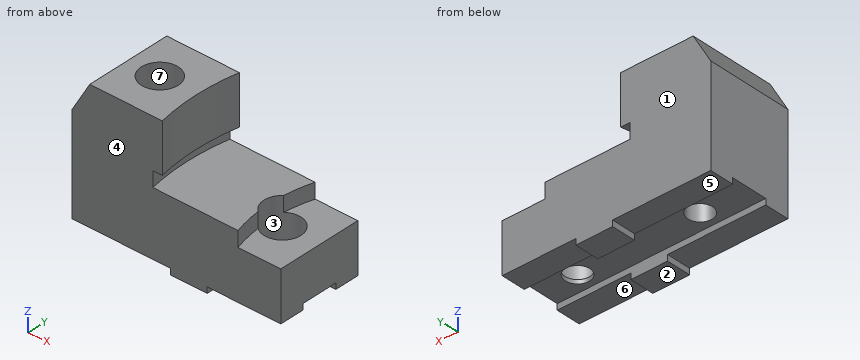
from build123d import *

# Parameters (mm, degrees)
F0_W                   = 107.95
F0_H                   = 69.85
F1_DEPTH               = 44.45
F2_W                   = 50.8254
F2_H                   = 3.048
F2_W_2                 = 38.1
F3_DEPTH               = 66.64201
F3_DEPTH_BACK          = 161
F4_W                   = 19.1008
F4_H                   = 3.048
F4_H_2                 = 17.1056788669
F5_DEPTH               = 107.951
F7_DEPTH               = 33.274
F9_W                   = 18.9599941809
F9_H                   = 7.874
F11_W                  = 28.8704986477
F11_H                  = 14.4021337534
F12_ANGLE_BACK         = 30
F12_ANGLE              = 60
F15_D                  = 12.7
F15_CBORE_D            = 19.05
F15_CBORE_DEPTH        = 20.574
F15_ON_F14_D           = 12.7
F15_ON_F14_START       = 7.874
F15_ON_F14_CBORE_D     = 19.05
F15_ON_F14_CBORE_DEPTH = 20.574


# Not quite as in the source:
# - an extrude ends at something that could not be found from the text; its depth is read off the source's solid
# - a length typed as a fraction of an inch, garbled in the dataset ("3 / 203.2 mm" for 3/8 in), is restored


with BuildPart() as f1:
    # F0 (on Front) → F1 (new body)
    with BuildSketch(Plane.XZ):
        with Locations((0.967470929, 9.7001004595)):
            Rectangle(F0_W, F0_H)
    extrude(amount=F1_DEPTH)

    # F2 (on face) → F3 (cut, two sides)
    with BuildSketch(Plane.XZ.offset(44.45)) as f3_sk:
        with Locations((-27.594829071, -23.7008995405)):
            Rectangle(F2_W, F2_H)
        with Locations((35.892470929, -23.7008995405)):
            Rectangle(F2_W_2, F2_H)
        Polygon((-53.007529071, 44.6251004595), (-43.9154170318, 44.6251004595), (-53.007529071, 49.8744337929), (-64.4665259088, 30.026869066), (-53.007529071, 28.8771004595), align=None)
        Polygon((-53.007529071, 28.8771004595), (-43.9154170318, 44.6251004595), (-53.007529071, 44.6251004595), align=None)
    extrude(amount=-F3_DEPTH, mode=Mode.SUBTRACT)
    extrude(f3_sk.sketch, amount=F3_DEPTH_BACK, mode=Mode.SUBTRACT)

    # F4 (on face) → F5 (cut, through all)
    with BuildSketch(Plane.YZ.offset(54.942470929)):
        with Locations((-22.1996, -20.6528995405)):
            Rectangle(F4_W, F4_H)
        with Locations((-22.1996, -30.7297389739)):
            Rectangle(F4_W, F4_H_2)
    extrude(amount=-F5_DEPTH, mode=Mode.SUBTRACT)

    # F6 (on face) → F7 (cut)
    with BuildSketch(Plane.XY.offset(44.6251004595)):
        with BuildLine():
            Line((84.230268681, 4.7385622747), (-0.8366582079, 19.0712375092))
            ThreePointArc((-0.8366582079, 19.0712375092), (-8.5367916359, -24.4021880093), (0.8136185269, -67.5507755982))
            Line((0.8136185269, -67.5507755982), (81.3293292463, -56.9063611329))
            Line((81.3293292463, -56.9063611329), (105.742470929, -22.225))
            Line((105.742470929, -22.225), (84.230268681, 4.7385622747))
        make_face()
    extrude(amount=-F7_DEPTH, mode=Mode.SUBTRACT)

    # F9 (on offset) → F10 (revolve, cut)
    with BuildSketch(Plane.XZ.offset(22.225)):
        with Locations((-3.9035319805, 15.2881004595)):
            Rectangle(F9_W, F9_H)
    revolve(axis=Axis((105.742470929, -22.225, 44.6251004595), (0, 0, 1)), mode=Mode.SUBTRACT)

    # F11 (on offset) → F12 (revolve, cut)
    with BuildSketch(Plane.XZ.offset(22.225), mode=Mode.PRIVATE) as f12_sk:
        with Locations((43.9777202529, 10.6781673362)):
            Rectangle(F11_W, F11_H)
    revolve(f12_sk.sketch.rotate(Axis((105.742470929, -22.225, 44.6251004595), (0, 0, -1)), -F12_ANGLE_BACK), axis=Axis((105.742470929, -22.225, 44.6251004595), (0, 0, -1)), revolution_arc=F12_ANGLE, mode=Mode.SUBTRACT)

    # F15 (through all)
    with Locations(Plane.XY.offset(44.6251004595)):
        with Locations((-27.607529071, -22.225)):
            CounterBoreHole(F15_D / 2, F15_CBORE_D / 2, F15_CBORE_DEPTH)

    # F15 on F14 (through all)
    # its depths count from where the whole tool has entered the part; down to there all is cleared
    with Locations(Plane.XY.offset(11.3511004595).offset(-F15_ON_F14_START)):
        with Locations((35.892470929, -22.225)):
            CounterBoreHole(F15_ON_F14_D / 2, F15_ON_F14_CBORE_D / 2, F15_ON_F14_CBORE_DEPTH)


solid = f1.part
Geometry check sheet. Reference: the model listing, model coordinates, mm. Face numbers are marked on the shaded views. A direction names the side the tool comes from. Give positions to 0.01 mm unless a question says otherwise; leave off trailing zeros. Order: outer loops, then holes, each group sorted by start corner. A loop starts at its lowest first (then second) coordinate and runs counter-clockwise, first axis right, second up. Notation, with made-up numbers: M 25,57.5 L 56,57.5 A14 ccw 56,64.5 Z; hole C 75,-36 d1. An arc over 180 degrees is marked long. Use a Markdown table: item, result.
Item 1: Section check C-C (z = 21). Record the cut outline in (x, y) (3 decimals), and give its area (3 significant figures).
Answers follow:
| item | result |
|---|---|
| outline | M -53.008,-44.45 L -6.376,-44.45 A114.3 cw -6.376,0 L -53.008,0 Z; hole C -27.608,-22.225 d12.7 |
| area | 1,880 mm2 |
Item 2: Section check D-D (x = 38.5). Record the cut outline in (y, z).
Answers follow:
| item | result |
|---|---|
| outline | M -44.45,-22.18 L -31.75,-22.18 L -31.75,-19.13 L -28.01,-19.13 L -28.01,-17.1 L -31.39,-17.1 L -31.39,3.48 L -44.45,3.48 Z; M -16.44,-19.13 L -12.65,-19.13 L -12.65,-22.18 L 0,-22.18 L 0,3.48 L -13.06,3.48 L -13.06,-17.1 L -16.44,-17.1 Z |
Item 3: Tool access check on the marked faces 5, 6 and 7. Record the directions out of +Z, -Z, +X, -X, +Y, -Y that give a thin tool (end or side, any length) a straight path to the whole face; none if there is none.
Answers follow:
| item | result |
|---|---|
| face 5 | -Z, -X, +Y, -Y |
| face 6 | -Z, +X, +Y, -Y |
| face 7 | +Z |
Item 4: Depth check by flat-ended pin: P1, Ø25, axis at x = 35.89, y = -22.22, coming from the -Z side; P2, Ø3, axis at x = -9, y = -26.5, coming from the -Z side; P3, Ø1.5, axis at y = -6.5, z = -23.5, coming from the -X side; P4, Ø15, axis at x = -31.5, y = -25, coming from the +Z side. Enter the tip coordinate at first touch or a pass-through.
Answers follow:
| item | result |
|---|---|
| P1 | stops at z = -22.18 |
| P2 | stops at z = -19.13 |
| P3 | stops at x = -2.18 |
| P4 | stops at z = 44.63 |
Item 5: Section check B-B (x = -40). Record the cut outline in (y, z).
Answers follow:
| item | result |
|---|---|
| outline | M -44.45,-22.18 L -31.75,-22.18 L -31.75,-19.13 L -12.65,-19.13 L -12.65,-22.18 L 0,-22.18 L 0,44.63 L -44.45,44.63 Z |
Item 6: Section check A-A (y = -26). Record the cut outline in (x, z).
Answers follow:
| item | result |
|---|---|
| outline | M -53.01,-19.13 L -32.71,-19.13 L -32.71,24.05 L -36.35,24.05 L -36.35,44.63 L -43.92,44.63 L -53.01,28.88 Z; M -22.5,-19.13 L 30.79,-19.13 L 30.79,-17.1 L 27.15,-17.1 L 27.15,11.35 L -13.32,11.35 L -13.32,19.23 L -8.5,19.23 L -8.5,44.63 L -18.86,44.63 L -18.86,24.05 L -22.5,24.05 Z; M 41,-19.13 L 54.94,-19.13 L 54.94,3.48 L 44.64,3.48 L 44.64,-17.1 L 41,-17.1 Z |
Item 7: Draft check along Y on the marked faces 1, 2, 3 and 4. Enter one of: +Y half, -Y half, draft (parallel to the pull), parting line (faces both ways), or undercut.
Answers follow:
| item | result |
|---|---|
| face 1 | +Y half |
| face 2 | draft |
| face 3 | undercut |
| face 4 | -Y half |
Item 8: Material ranges on line 1 along Z through (x, y) = (-38, -29.5); line 2 along Z through (x, y) = (10, -22.5); line 3 along Y through (x, z) = (-22, -4.5), recorded low to high.
Answers follow:
| item | result |
|---|---|
| line 1 | z = -19.13 to 44.63 |
| line 2 | z = -19.13 to 11.35 |
| line 3 | y = -44.45 to -25.2, -19.25 to 0 |
